Verification items for the finished model (mm, model axes). Round coordinates to 2 decimals unless told otherwise and drop trailing zeros. Order: outer loops, then holes, each group sorted by start corner. A loop starts at its lowest first (then second) coordinate and runs counter-clockwise, first axis right, second up. Notation, with made-up numbers: (31, -17) -> (60, -17) arc R25 cw to (60, 1) -> close; hole circle Ø1 at (47, -17). An arc over 180 degrees is marked (long way). Put each result on its own line as item: value.
from build123d import *

# Parameters (mm, degrees)
SKETCH_1_W          = 17.893001423
SKETCH_1_H          = 11.620982588
SKETCH_1_H_2        = 11.620982589
EXTRUDE_1_DEPTH     = 1
SKETCH_2_R          = 1.5
CUT_EXTRUDE_1_DEPTH = 10
CHAMFER_1_SIZE      = 1
SKETCH_3_R          = 1.5
CUT_EXTRUDE_2_DEPTH = 10
CHAMFER_2_SIZE      = 1


with BuildPart() as part:
    # Эскиз1 → Бобышка-Вытянуть1 (new body)
    with BuildSketch(Plane(origin=(0, 0, 0), x_dir=(1, 0, 0), z_dir=(0, 1, 0))):
        Polygon((49.933797981, 26), (18.809932441, 26), (18.809932441, 48), (15, 48), (-48.959081244, 48), (-48.959081244, -48), (15, -48), (18.809932441, -48), (18.809932441, -26), (49.933797981, -26), align=None)
        with Locations((-36.319088007, -31.12001489)):
            Rectangle(SKETCH_1_W, SKETCH_1_H, mode=Mode.SUBTRACT)
        with Locations((-36.319088007, 31.12001489)):
            Rectangle(SKETCH_1_W, SKETCH_1_H_2, mode=Mode.SUBTRACT)
    extrude(amount=EXTRUDE_1_DEPTH)

    # Эскиз2 → Вырез-Вытянуть1 (cut)
    with BuildSketch(Plane(origin=(0, 1, 0), x_dir=(1, 0, 0), z_dir=(0, 1, 0))):
        with Locations(Location((46.183797981, -14.4, 0), (0, 0, 270))):
            Circle(SKETCH_2_R)
        with Locations(Location((18.683797981, -14.4, 0), (0, 0, 270))):
            Circle(SKETCH_2_R)
        with Locations(Location((18.683797981, -4.4, 0), (0, 0, 270))):
            Circle(SKETCH_2_R)
        with Locations(Location((46.183797981, -4.4, 0), (0, 0, 270))):
            Circle(SKETCH_2_R)
        with Locations(Location((18.683797981, 5.6, 0), (0, 0, 270))):
            Circle(SKETCH_2_R)
        with Locations(Location((46.183797981, 5.6, 0), (0, 0, 270))):
            Circle(SKETCH_2_R)
        with Locations(Location((18.683797981, 15.6, 0), (0, 0, 270))):
            Circle(SKETCH_2_R)
        with Locations(Location((46.183797981, 15.6, 0), (0, 0, 270))):
            Circle(SKETCH_2_R)
    extrude(amount=-CUT_EXTRUDE_1_DEPTH, mode=Mode.SUBTRACT)

    # Фаска1
    chamfer_1_edges = [part.edges().sort_by_distance(p)[0] for p in [
        (46.183797981, 0, -7.1),
        (18.683797981, 0, 2.9),
        (46.183797981, 0, 2.9),
        (18.683797981, 0, 12.9),
        (18.683797981, 0, -17.1),
        (46.183797981, 0, -17.1),
        (18.683797981, 0, -7.1),
        (46.183797981, 0, 12.9),
    ]]
    chamfer(chamfer_1_edges, length=CHAMFER_1_SIZE - 0.0001)  # a hair under: the kernel refuses the full size

    # Эскиз3 → Вырез-Вытянуть2 (cut)
    with BuildSketch(Plane(origin=(0, 1, 0), x_dir=(1, 0, 0), z_dir=(0, 1, 0))):
        with Locations(Location((5.923569009, 32.746976788, 0), (0, 0, 270))):
            Circle(SKETCH_3_R)
        with Locations(Location((-2.726430991, 32.746976788, 0), (0, 0, 270))):
            Circle(SKETCH_3_R)
        with Locations(Location((-2.726430991, -35.660220789, 0), (0, 0, 270))):
            Circle(SKETCH_3_R)
        with Locations(Location((5.923569009, -35.660220789, 0), (0, 0, 270))):
            Circle(SKETCH_3_R)
    extrude(amount=-CUT_EXTRUDE_2_DEPTH, mode=Mode.SUBTRACT)

    # Фаска2
    chamfer_2_edges = [part.edges().sort_by_distance(p)[0] for p in [
        (5.923569009, 0, 34.160220789),
        (-2.726430991, 0, 34.160220789),
        (-2.726430991, 0, -34.246976788),
        (5.923569009, 0, -34.246976788),
    ]]
    chamfer(chamfer_2_edges, length=CHAMFER_2_SIZE - 0.0001)  # a hair under: the kernel refuses the full size


solid = part.part
Item 1: Gauge pin test, flat end, axial feed: pin 1 Ø1.8 at (x, z) = (5.92, -32.75) entering from -Y. Record the tip position at first contact, or that the pin passes through.
Check sheet entries:
pin 1: passes through
Item 2: Section check D-D on x = 32.5. Record the boundary of the cut face in (y, z), then the cut area to 3 significant figures.
Check sheet entries:
outline: (0, -26) -> (1, -26) -> (1, 26) -> (0, 26) -> close
area: 52.0 mm^2
Item 3: Section check B-B on z = -15.6. State how many separate pieces and enclosed holes the cut face has, then the cut area to 3 significant figures.
Check sheet entries:
separate pieces: 3
enclosed holes: 0
area: 90.9 mm^2
Item 4: Material ranges on L1, parallel to Z at x = -41, y = 0.25; L2, parallel to X at y = 0.9, z = -29.5; L3, parallel to X at y = 0.85, z = -16, recorded low to high. Write a range as [from, to].
Check sheet entries:
L1: z = [-48, -36.93], [-25.31, 25.31], [36.93, 48]
L2: x = [-48.96, -45.27], [-27.37, 18.81]
L3: x = [-48.96, 17.08], [20.28, 44.58], [47.78, 49.93]
Item 5: Section check A-A on x = -32. Record the boundary of the cut face in (y, z).
Check sheet entries:
outline: (0, -48) -> (1, -48) -> (1, -36.93) -> (0, -36.93) -> close; (0, -25.31) -> (1, -25.31) -> (1, 25.31) -> (0, 25.31) -> close; (0, 36.93) -> (1, 36.93) -> (1, 48) -> (0, 48) -> close
